```python
from build123d import *

# Parameters (mm, degrees)
F0_W     = 250
F0_H     = 101.666841656
F1_DEPTH = 50


with BuildPart() as f1:
    # F0 (on Front) → F1 (new body)
    with BuildSketch(Plane.XZ):
        with Locations((5.5693238974, 4.9150865525)):
            Rectangle(F0_W, F0_H)
        with BuildLine():
            Line((-79.1357593007, -8.4097307281), (-79.1357593007, -15.8393876627))
            Line((-79.1357593007, -15.8393876627), (-108.3243500131, -15.8393876627))
            Line((-108.3243500131, -15.8393876627), (-108.3243500131, -9.6982690156))
            Line((-108.3243500131, -9.6982690156), (-97.8424108938, 0.8933329367))
            add(Edge.make_bspline(
                [(-97.8424108938, 0.8933329367), (-93.181740492, 5.6636661714), (-91.7561236632, 7.5050879086)],
                knots=[0, 0, 0, 1, 1, 1], degree=2))
            add(Edge.make_bspline(
                [(-91.7561236632, 7.5050879086), (-90.3305068344, 9.3465096458), (-89.6999455448, 10.9183435852)],
                knots=[0, 0, 0, 1, 1, 1], degree=2))
            add(Edge.make_bspline(
                [(-89.6999455448, 10.9183435852), (-89.0693842551, 12.4901775246), (-89.0693842551, 14.1716742971)],
                knots=[0, 0, 0, 1, 1, 1], degree=2))
            add(Edge.make_bspline(
                [(-89.0693842551, 14.1716742971), (-89.0693842551, 16.6847808863), (-90.4584468062, 17.9139184726)],
                knots=[0, 0, 0, 1, 1, 1], degree=2))
            add(Edge.make_bspline(
                [(-90.4584468062, 17.9139184726), (-91.8475093573, 19.143056059), (-94.1595674194, 19.143056059)],
                knots=[0, 0, 0, 1, 1, 1], degree=2))
            add(Edge.make_bspline(
                [(-94.1595674194, 19.143056059), (-96.5812883145, 19.143056059), (-98.8659306683, 18.0281505903)],
                knots=[0, 0, 0, 1, 1, 1], degree=2))
            add(Edge.make_bspline(
                [(-98.8659306683, 18.0281505903), (-101.1505730221, 16.9132451216), (-103.6362639031, 14.8570670032)],
                knots=[0, 0, 0, 1, 1, 1], degree=2))
            Line((-103.6362639031, 14.8570670032), (-108.4340128461, 20.5412571795))
            add(Edge.make_bspline(
                [(-108.4340128461, 20.5412571795), (-105.3543149531, 23.1731651711), (-103.3255525429, 24.2560856468)],
                knots=[0, 0, 0, 1, 1, 1], degree=2))
            add(Edge.make_bspline(
                [(-103.3255525429, 24.2560856468), (-101.2967901327, 25.3390061225), (-98.8979156612, 25.9238745651)],
                knots=[0, 0, 0, 1, 1, 1], degree=2))
            add(Edge.make_bspline(
                [(-98.8979156612, 25.9238745651), (-96.4990411897, 26.5087430077), (-93.5290061298, 26.5087430077)],
                knots=[0, 0, 0, 1, 1, 1], degree=2))
            add(Edge.make_bspline(
                [(-93.5290061298, 26.5087430077), (-89.61769842, 26.5087430077), (-86.6202476518, 25.0831261789)],
                knots=[0, 0, 0, 1, 1, 1], degree=2))
            add(Edge.make_bspline(
                [(-86.6202476518, 25.0831261789), (-83.6227968836, 23.6575093501), (-81.9641465347, 21.0850020597)],
                knots=[0, 0, 0, 1, 1, 1], degree=2))
            add(Edge.make_bspline(
                [(-81.9641465347, 21.0850020597), (-80.3054961859, 18.5124947693), (-80.3054961859, 15.204332641)],
                knots=[0, 0, 0, 1, 1, 1], degree=2))
            add(Edge.make_bspline(
                [(-80.3054961859, 15.204332641), (-80.3054961859, 12.3165447058), (-81.3198773909, 9.7897302624)],
                knots=[0, 0, 0, 1, 1, 1], degree=2))
            add(Edge.make_bspline(
                [(-81.3198773909, 9.7897302624), (-82.334258596, 7.2629158191), (-84.4635452698, 4.608161404)],
                knots=[0, 0, 0, 1, 1, 1], degree=2))
            add(Edge.make_bspline(
                [(-84.4635452698, 4.608161404), (-86.5928319436, 1.9534069888), (-91.9571721903, -2.9631433566)],
                knots=[0, 0, 0, 1, 1, 1], degree=2))
            Line((-91.9571721903, -2.9631433566), (-97.3306510065, -8.0167722432))
            Line((-97.3306510065, -8.0167722432), (-97.3306510065, -8.4097307281))
            Line((-97.3306510065, -8.4097307281), (-79.1357593007, -8.4097307281))
        make_face(mode=Mode.SUBTRACT)
        with BuildLine():
            add(Edge.make_bspline(
                [(-49.6775807906, 21.0895713444), (-45.9810294621, 15.6064296953), (-45.9810294621, 5.0331048818)],
                knots=[0, 0, 0, 1, 1, 1], degree=2))
            add(Edge.make_bspline(
                [(-45.9810294621, 5.0331048818), (-45.9810294621, -5.8966241389), (-49.5633486729, -11.1558708374)],
                knots=[0, 0, 0, 1, 1, 1], degree=2))
            add(Edge.make_bspline(
                [(-49.5633486729, -11.1558708374), (-53.1456678837, -16.4151175359), (-60.6027405265, -16.4151175359)],
                knots=[0, 0, 0, 1, 1, 1], degree=2))
            add(Edge.make_bspline(
                [(-60.6027405265, -16.4151175359), (-67.831348934, -16.4151175359), (-71.5004845542, -10.9868073032)],
                knots=[0, 0, 0, 1, 1, 1], degree=2))
            add(Edge.make_bspline(
                [(-71.5004845542, -10.9868073032), (-75.1696201745, -5.5584970705), (-75.1696201745, 5.0331048818)],
                knots=[0, 0, 0, 1, 1, 1], degree=2))
            add(Edge.make_bspline(
                [(-75.1696201745, 5.0331048818), (-75.1696201745, 16.0907738743), (-71.5964395331, 21.3317434339)],
                knots=[0, 0, 0, 1, 1, 1], degree=2))
            add(Edge.make_bspline(
                [(-71.5964395331, 21.3317434339), (-68.0232588917, 26.5727129936), (-60.6027405265, 26.5727129936)],
                knots=[0, 0, 0, 1, 1, 1], degree=2))
            add(Edge.make_bspline(
                [(-60.6027405265, 26.5727129936), (-53.374132119, 26.5727129936), (-49.6775807906, 21.0895713444)],
                knots=[0, 0, 0, 1, 1, 1], degree=2))
        make_face(mode=Mode.SUBTRACT)
        with BuildLine():
            Line((-19.7350581014, 25.9147359957), (-19.7350581014, -15.8393876627))
            Line((-19.7350581014, -15.8393876627), (-28.5629161566, -15.8393876627))
            Line((-28.5629161566, -15.8393876627), (-28.5629161566, 8.3229898713))
            Line((-28.5629161566, 8.3229898713), (-28.4715304624, 12.2891289975))
            Line((-28.4715304624, 12.2891289975), (-28.3344519212, 16.6299494698))
            add(Edge.make_bspline(
                [(-28.3344519212, 16.6299494698), (-30.5277085808, 14.4366928101), (-31.3867341059, 13.751300104)],
                knots=[0, 0, 0, 1, 1, 1], degree=2))
            Line((-31.3867341059, 13.751300104), (-36.1844830489, 9.8948238107))
            Line((-36.1844830489, 9.8948238107), (-40.4430563964, 15.204332641))
            Line((-40.4430563964, 15.204332641), (-26.9910822171, 25.9147359957))
            Line((-26.9910822171, 25.9147359957), (-19.7350581014, 25.9147359957))
        make_face(mode=Mode.SUBTRACT)
        with BuildLine():
            add(Edge.make_bspline(
                [(-6.5892259975, -8.0167722432), (-8.458063443, -3.9044160064), (-8.458063443, 1.8985755723)],
                knots=[0, 0, 0, 1, 1, 1], degree=2))
            add(Edge.make_bspline(
                [(-8.458063443, 1.8985755723), (-8.458063443, 14.2904756995), (-3.2170938833, 20.3447779371)],
                knots=[0, 0, 0, 1, 1, 1], degree=2))
            add(Edge.make_bspline(
                [(-3.2170938833, 20.3447779371), (2.0238756764, 26.3990801747), (12.4783990874, 26.3990801747)],
                knots=[0, 0, 0, 1, 1, 1], degree=2))
            add(Edge.make_bspline(
                [(12.4783990874, 26.3990801747), (16.0424411594, 26.3990801747), (18.0712035696, 25.9695674122)],
                knots=[0, 0, 0, 1, 1, 1], degree=2))
            Line((18.0712035696, 25.9695674122), (18.0712035696, 18.9145918236))
            add(Edge.make_bspline(
                [(18.0712035696, 18.9145918236), (15.5306812721, 19.4903216967), (13.0449903912, 19.4903216967)],
                knots=[0, 0, 0, 1, 1, 1], degree=2))
            add(Edge.make_bspline(
                [(13.0449903912, 19.4903216967), (8.5031213918, 19.4903216967), (5.6336105954, 18.1195362845)],
                knots=[0, 0, 0, 1, 1, 1], degree=2))
            add(Edge.make_bspline(
                [(5.6336105954, 18.1195362845), (2.764099799, 16.7487508722), (1.3384829702, 14.0620114641)],
                knots=[0, 0, 0, 1, 1, 1], degree=2))
            add(Edge.make_bspline(
                [(1.3384829702, 14.0620114641), (-0.0871338586, 11.375272056), (-0.3430138022, 6.4404445717)],
                knots=[0, 0, 0, 1, 1, 1], degree=2))
            Line((-0.3430138022, 6.4404445717), (0.0225289744, 6.4404445717))
            add(Edge.make_bspline(
                [(0.0225289744, 6.4404445717), (2.8554854932, 11.2930249312), (9.078851265, 11.2930249312)],
                knots=[0, 0, 0, 1, 1, 1], degree=2))
            add(Edge.make_bspline(
                [(9.078851265, 11.2930249312), (14.6716557471, 11.2930249312), (17.8427393342, 7.7792449911)],
                knots=[0, 0, 0, 1, 1, 1], degree=2))
            add(Edge.make_bspline(
                [(17.8427393342, 7.7792449911), (21.0138229213, 4.2654650509), (21.0138229213, -1.9304850127)],
                knots=[0, 0, 0, 1, 1, 1], degree=2))
            add(Edge.make_bspline(
                [(21.0138229213, -1.9304850127), (21.0138229213, -8.6107792552), (17.2441630375, -12.5129483955)],
                knots=[0, 0, 0, 1, 1, 1], degree=2))
            add(Edge.make_bspline(
                [(17.2441630375, -12.5129483955), (13.4745031537, -16.4151175359), (6.7942089111, -16.4151175359)],
                knots=[0, 0, 0, 1, 1, 1], degree=2))
            add(Edge.make_bspline(
                [(6.7942089111, -16.4151175359), (2.170092787, -16.4151175359), (-1.2751478826, -14.272123008)],
                knots=[0, 0, 0, 1, 1, 1], degree=2))
            add(Edge.make_bspline(
                [(-1.2751478826, -14.272123008), (-4.7203885521, -12.1291284801), (-6.5892259975, -8.0167722432)],
                knots=[0, 0, 0, 1, 1, 1], degree=2))
        make_face(mode=Mode.SUBTRACT)
        Polygon((38.8340332811, 25.9147359957), (46.7480343947, 25.9147359957), (31.1759121111, -15.8393876627), (23.2710495669, -15.8393876627), align=None, mode=Mode.SUBTRACT)
        with BuildLine():
            Line((71.1937075806, 25.9147359957), (71.1937075806, -15.8393876627))
            Line((71.1937075806, -15.8393876627), (62.3658495254, -15.8393876627))
            Line((62.3658495254, -15.8393876627), (62.3658495254, 8.3229898713))
            Line((62.3658495254, 8.3229898713), (62.4572352196, 12.2891289975))
            Line((62.4572352196, 12.2891289975), (62.5943137608, 16.6299494698))
            add(Edge.make_bspline(
                [(62.5943137608, 16.6299494698), (60.4010571011, 14.4366928101), (59.5420315761, 13.751300104)],
                knots=[0, 0, 0, 1, 1, 1], degree=2))
            Line((59.5420315761, 13.751300104), (54.7442826331, 9.8948238107))
            Line((54.7442826331, 9.8948238107), (50.4857092856, 15.204332641))
            Line((50.4857092856, 15.204332641), (63.9376834649, 25.9147359957))
            Line((63.9376834649, 25.9147359957), (71.1937075806, 25.9147359957))
        make_face(mode=Mode.SUBTRACT)
        Polygon((96.1511406537, -15.8393876627), (86.893769836, -15.8393876627), (102.5755549526, 18.4302476446), (81.98635806, 18.4302476446), (81.98635806, 25.8599045792), (111.9425886033, 25.8599045792), (111.9425886033, 20.3127929441), align=None, mode=Mode.SUBTRACT)
    extrude(amount=F1_DEPTH)


solid = f1.part
```
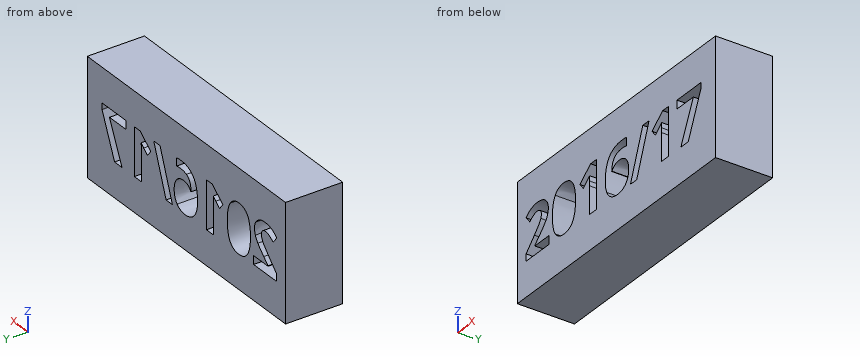
Here's how the part is built. I have some questions about the finished solid (model axes, mm). Give positions to 0.01 mm unless a question says otherwise; leave off trailing zeros. Order: outer loops, then holes, each group sorted by start corner. A loop starts at its lowest first (then second) coordinate and runs counter-clockwise, first axis right, second up. Notation, with made-up numbers: (40.25, 60) - (60.25, 60) arc R24 cw to (60.25, 89) - close; hole circle Ø6 at (-25.5, -18). An arc over 180 degrees is marked (long way). Answer as a JSON object with one key per item and string values. Group by question number.
Item 1: Please list where these lines run through material, in increasing order: probe 1 along Z at (x, y) = (-102.5, -35); probe 2 along Z at (x, y) = (-89, -23.5); probe 3 along Z at (x, y) = (-32.5, -20.5).
Item 2: If we section it at A-A on x = 91: Please give me the cut outline in (y, z).
Item 3: If we section it at B-B on y = -18: Give the number of separate pieces and of enclosed holes in the cut face, and give its area (3 significant figures).
Item 4: For P1, Ø5, axis at x = -90, z = 23, coming from the -Y side, with a flat end and sliding along its axis, tell me the tip position at first contact or that it passes through.
Result set:
{
 "1": {"probe 1": "-45.92 to -15.84, -3.81 to 15.76, 24.67 to 55.75", "probe 2": "-45.92 to -15.84, -8.41 to -0.19, 25.95 to 55.75", "probe 3": "-45.92 to 12.86, 21.53 to 55.75"},
 "2": {"outline": "(-50, -45.92) - (0, -45.92) - (0, -15.84) - (-50, -15.84) - close; (-50, -6.87) - (0, -6.87) - (0, 18.43) - (-50, 18.43) - close; (-50, 25.86) - (0, 25.86) - (0, 55.75) - (-50, 55.75) - close"},
 "3": {"separate pieces": "1", "enclosed holes": "7", "area": "21,100 mm²"},
 "4": {"P1": "through"}
}
